from build123d import *

# Parameters (mm, degrees)
F0_W          = 50
F0_H          = 100
F1_DEPTH      = 10
F3_DEPTH      = 50
F3_DEPTH_BACK = 30
F4_W          = 5.3
F4_H          = 3.3
F5_DEPTH      = 1.5
F6_R          = 6
F7_DEPTH      = 4
F8_R          = 3.15
F9_DEPTH      = 6


with BuildPart() as f1:
    # F0 (on Top) → F1 (new body)
    with BuildSketch(Plane.XY):
        Rectangle(F0_W, F0_H)
    extrude(amount=F1_DEPTH)

    # F2 (on Front) → F3 (cut, two sides)
    with BuildSketch(Plane.XZ) as f3_sk:
        Polygon((-5.1, 0), (0, 0), (5.1, 0), (13.2, 8.1), (0, 8.1), (-13.2, 8.1), align=None)
    extrude(amount=-F3_DEPTH, mode=Mode.SUBTRACT)
    extrude(f3_sk.sketch, amount=F3_DEPTH_BACK, mode=Mode.SUBTRACT)

    # F4 (on face) → F5 (cut)
    with BuildSketch(Plane.XY.offset(10)):
        with Locations((-10.45, 38.55)):
            Rectangle(F4_W, F4_H)
        with Locations((10.45, 38.55)):
            Rectangle(F4_W, F4_H)
    extrude(amount=-F5_DEPTH, mode=Mode.SUBTRACT)

    # F6 (on face) → F7 (cut)
    with BuildSketch(Plane(origin=(0, 0, 0), x_dir=(1, 0, 0), z_dir=(0, 0, -1))):
        with Locations((0, 37.2307598591)):
            Circle(F6_R)
    extrude(amount=-F7_DEPTH, mode=Mode.SUBTRACT)

    # F8 (on face) → F9 (cut, through all)
    with BuildSketch(Plane(origin=(0, 0, 4), x_dir=(1, 0, 0), z_dir=(0, 0, -1))):
        with Locations((0, 37.2307598591)):
            Circle(F8_R)
    extrude(amount=-F9_DEPTH, mode=Mode.SUBTRACT)


solid = f1.part
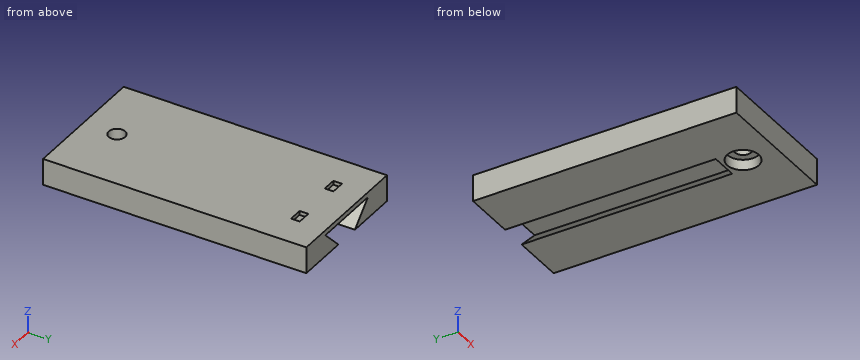
Part model, mm, in its own coordinate system. Round coordinates to 2 decimals unless told otherwise and drop trailing zeros. Write each loop counter-clockwise with the first axis right and the second up, starting at its lowest first coordinate (ties: lowest second). Pieces come first, ordered by that corner, then holes. Notation, with made-up numbers: M -20.5,67 L -1.5,67 A29 cw -1.5,89 Z; hole C 31.25,-10.5 d1. An arc over 180 degrees is marked long. Return JSON: item names as keys, results as strings. Group by question number.
(1) Pin check, flat tips, straight feed: pin 1 Ø4 at (x, z) = (-1.5, 4) entering from +Y; pin 2 Ø6 at (x, y) = (-0.5, -38.5) entering from -Z; pin 3 Ø1.6 at (x, y) = (-10.5, 39) entering from +Z. Stop position of each tip, or through.
(2) Saw through at B-B on y = 19. Write the cut outline in (x, z), then the cut area to 3 significant figures.
(3) Saw through at C-C on x = -11. Write the cut outline in (y, z), then the cut area to 3 significant figures.
(4) Saw through at D-D on z = 7. Write the cut outline in (x, y), then the cut area to 3 significant figures.
(5) Drill centre lines: probe 1 along Y at (x, z) = (0, 0.8); probe 2 along Y at (x, z) = (0, 8.4); probe 3 along Z at (x, y) = (-1.5, 16.5). Where is each one in solid material? Low to high.
(6) Saw through at A-A on x = 0. Write the cut outline in (y, z).
Returned:
{
 "1": {"pin 1": "y = -30", "pin 2": "z = 4", "pin 3": "z = 8.5"},
 "2": {"outline": "M -25,0 L -5.1,0 L -13.2,8.1 L 13.2,8.1 L 5.1,0 L 25,0 L 25,10 L -25,10 Z", "area": "352 mm²"},
 "3": {"outline": "M -50,0 L 50,0 L 50,5.9 L -30,5.9 L -30,8.1 L 50,8.1 L 50,10 L 40.2,10 L 40.2,8.5 L 36.9,8.5 L 36.9,10 L -50,10 Z", "area": "819 mm²"},
 "4": {"outline": "M -25,-50 L 25,-50 L 25,50 L 12.1,50 L 12.1,-30 L -12.1,-30 L -12.1,50 L -25,50 Z; hole C 0,-37.23 d6.3", "area": "3,030 mm²"},
 "5": {"probe 1": "-50 to -43.23, -31.23 to -30", "probe 2": "-50 to -40.38, -34.08 to 50", "probe 3": "8.1 to 10"},
 "6": {"outline": "M -50,0 L -43.23,0 L -43.23,4 L -40.38,4 L -40.38,10 L -50,10 Z; M -34.08,4 L -31.23,4 L -31.23,0 L -30,0 L -30,8.1 L 50,8.1 L 50,10 L -34.08,10 Z"}
}
